Geometry: final body of the model. Coordinates: model frame, mm. A direction names the side the tool comes from. Give positions to 0.01 mm unless a question says otherwise; leave off trailing zeros. Write each loop counter-clockwise with the first axis right and the second up, starting at its lowest first coordinate (ties: lowest second). Pieces come first, ordered by that corner, then holes.
Autodesk Inventor part; units mm, degrees
ref_plane "YZ Plane" through (0, 0, 0) normal (1, 0, 0) x (0, 1, 0)
ref_plane "XZ Plane" through (0, 0, 0) normal (0, 1, 0) x (-1, 0, 0)
ref_plane "XY Plane" through (0, 0, 0) normal (0, 0, 1) x (1, 0, 0)
sketch "Sketch1" plane through (0, 0, 0) normal (0, 1, 0) x (-1, 0, 0)
  circle A0 centre (0, 0) radius 6.9215
  dimension "d0" = 13.843
extrude "Extrusion1" add sketch "Sketch1" along normal blind 13.843
hole "Hole2" at (0, 0, 0) direction (0, 1, 0) diameter 12.192 depth 3.175
hole "Hole1" at (0, 3.175, 0) direction (0, 1, 0) diameter 11.43 depth 9.144
sketch "Sketch2" plane through (0, 0, 0) normal (1, 0, 0) x (0, 1, 0)
  line L0 (13.843, -6.9215) -> (13.843, 6.9215)
  line L1 (13.843, 0) -> (7.493, 0)
  circle A0 centre (7.493, 0) radius 1.7399
  point P0 (0, 0)
  dimension "d21" = 6.35
  dimension "d22" = 3.4798
extrude "Extrusion2" cut sketch "Sketch2" along normal through all both and the other way through all
sketch "Workplane Control Sketch" plane through (0, 13.843, 0) normal (0, 1, 0) x (1, 0, 0)
  circle A0 centre (0, 0) radius 6.9215
  line L0 (0, 0) -> (4.89424, 4.89424)
  line L1 (0, 0) -> (0, 6.9215) construction
  dimension "d25" = 45
ref_plane "Work Plane1" through (4.89424, 13.843, -4.89424) normal (0.7071068, 0, -0.7071068) x (0, 1, 0)
sketch "Sketch4" plane through (4.89424, 13.843, -4.89424) normal (0.7071068, 0, -0.7071068) x (0, 1, 0)
  line L0 (0, 0) -> (-5.08, 0)
  circle A0 centre (-5.08, 0) radius 2.54
  point P0 (-13.843, 0)
  dimension "d26" = 5.08
  dimension "d27" = 5.08
extrude "Extrusion3" cut sketch "Sketch4" against normal up to next
properties part number "Piston" material "Aluminum 6061"
Q1. Section A-A on z = 0. Count the separate pieces of the cut face and the enclosed holes in it, plus the area to 3 significant figures.
Filled sheet:
separate pieces: 3
enclosed holes: 0
area: 40.0 mm2
Q2. Section C-C on y = 1. Output: boundary loops of the cut face in (x, z), plus the area to 3 significant figures.
Filled sheet:
outline: circle Ø13.84 at (0, 0); hole circle Ø12.19 at (0, 0)
area: 33.8 mm2
Q3. Access query for faces 5 (the flat face through (0, 13.843, 0)), 6 (the cylindrical face through (-3.862, 7.811, 4.212)). Directions: +Z, -Z, +X, -X, +Y, -Y. A direction counts if a zero-diameter tool reaches every point of the face in a straight line with its end or side. Return the directions, or none.
Filled sheet:
face 5: +Z, -Z, +X, -X, +Y
face 6: -Y
Q4. Section D-D on z = 4.5. Output: boundary loops of the cut face in (x, y) (3 decimals).
Filled sheet:
outline: (-5.259, 0) - (-4.112, 0) - (-4.112, 3.175) - (-3.523, 3.175) - (-3.523, 12.319) - (3.523, 12.319) - (3.523, 3.175) - (4.112, 3.175) - (4.112, 0) - (5.259, 0) - (5.259, 13.843) - (-5.259, 13.843) - close
Q5. Ray query, line 1 along X through (y, z) = (1.9, 0); line 2 along X through (y, z) = (9.5, 0) (1 decimal). Return the intervals inside material, ascending.
Filled sheet:
line 1: x = -6.92 to -6.1, 6.1 to 6.92
line 2: x = -6.9 to -5.7, 5.7 to 6.9
Q6. Pin query (flat end, axial travel): P1, Ø6, axis at x = 5, y = 6.5, coming from the -Z side; P2, Ø3.5, axis at x = 0.5, z = 1, coming from the -Y side. Return the tip coordinate at first contact, or that it passes through.
Filled sheet:
P1: stops at z = -6.63
P2: stops at y = 12.32
Q7. Pull-direction query (Z, two-part tool) for faces 1 (the cylindrical face through (-6.394, 6.825, 2.651)), 2 (the flat face through (-4, 0, -5)), 3 (the cylindrical face through (3.6, 11.1, -5)), 4 (the cylindrical face through (-6.044, 1.61, 0.794)); classes: released by +Z, released by -Z, zero draft, split by the parting line, or undercut.
Filled sheet:
face 1: split by the parting line
face 2: zero draft
face 3: undercut
face 4: undercut
